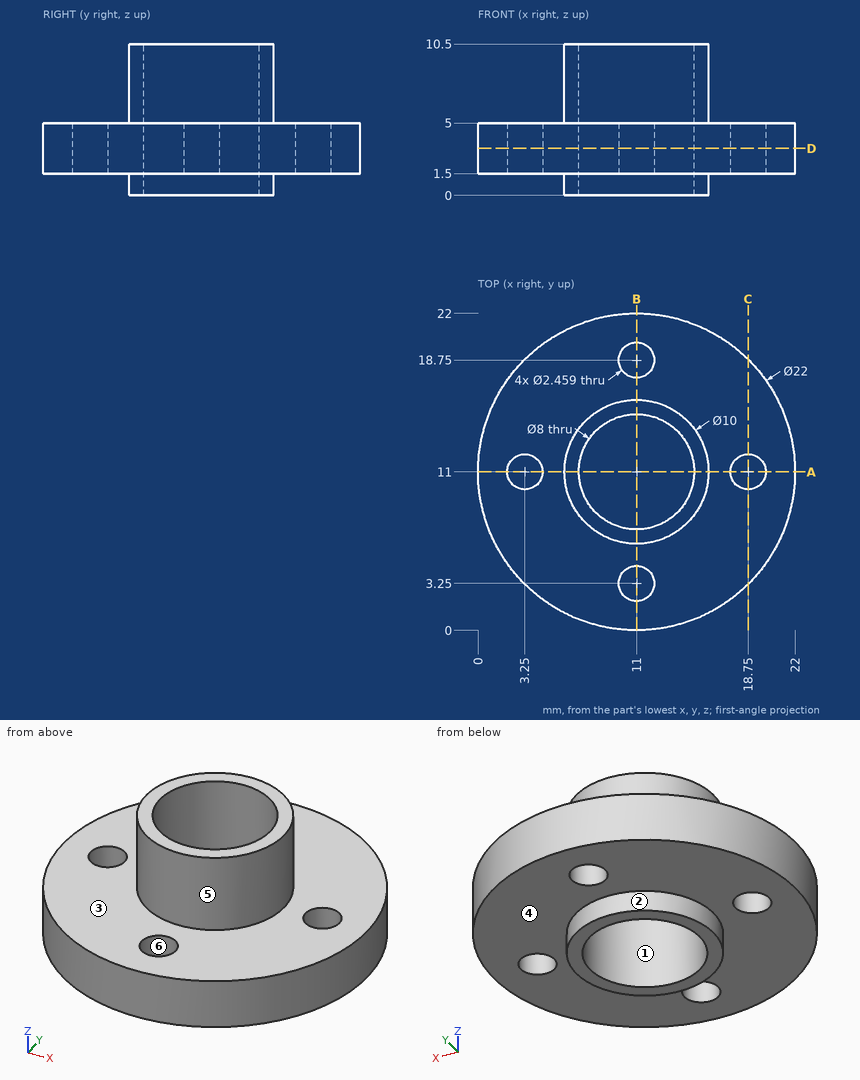
Geometry check sheet. Reference: drawing and pictorial views, mm from the part's lowest x, y, z. A direction names the side the tool comes from. Coordinates: 2 decimals unless noted, no trailing zeros. Write each loop counter-clockwise with the first axis right and the second up, starting at its lowest first coordinate (ties: lowest second). Pieces come first, ordered by that corner, then holes.
Item 1: Mould release check, pull along X, two halves, no side actions. Record for the marked faces 4, 5 and 6: released by +X, released by -X, zero draft, split by the parting line, or undercut.
Numbers:
face 4: zero draft
face 5: split by the parting line
face 6: undercut
Item 2: Access from +Z, -Z, +X, -X, +Y, -Y to the whole of each face (thin tool, end or side, straight path). Record for the marked faces 1, 2 and 3.
Numbers:
face 1: +Z, -Z
face 2: -Z
face 3: +Z
Item 3: Cross-section at D-D on z = 3.25. Record the boundary of the cut face in (x, y).
Numbers:
outline: circle Ø22 at (11, 11); hole circle Ø2.46 at (3.25, 11); hole circle Ø8 at (11, 11); hole circle Ø2.46 at (11, 3.25); hole circle Ø2.46 at (11, 18.75); hole circle Ø2.46 at (18.75, 11)
Item 4: Scan lines: probe 1 along X at (y, z) = (11, 3.7); probe 2 along Z at (x, y) = (18, 15.75); probe 3 along X at (y, z) = (11, 6.5). Record each from-to range of solid material in increasing order.
Numbers:
probe 1: x = 0 to 2.02, 4.48 to 7, 15 to 17.52, 19.98 to 22
probe 2: z = 1.5 to 5
probe 3: x = 6 to 7, 15 to 16
Item 5: Depth check by flat-ended pin: pin 1 Ø3 at (x, z) = (9, 8.5) entering from +Y; pin 2 Ø3 at (x, y) = (11, 3.25) entering from +Z; pin 3 Ø5 at (x, z) = (16, 4.5) entering from -Y. Enter the tip coordinate at first touch or a pass-through.
Numbers:
pin 1: stops at y = 15.97
pin 2: stops at z = 5
pin 3: stops at y = 0.29
Item 6: Cross-section at A-A on y = 11. Record the boundary of the cut face in (x, z), then the cut area to 3 significant figures.
Numbers:
outline: (0, 1.5) - (2.02, 1.5) - (2.02, 5) - (0, 5) - close; (4.48, 1.5) - (6, 1.5) - (6, 0) - (7, 0) - (7, 10.5) - (6, 10.5) - (6, 5) - (4.48, 5) - close; (15, 0) - (16, 0) - (16, 1.5) - (17.52, 1.5) - (17.52, 5) - (16, 5) - (16, 10.5) - (15, 10.5) - close; (19.98, 1.5) - (22, 1.5) - (22, 5) - (19.98, 5) - close
area: 45.8 mm2
Item 7: Cross-section at C-C on x = 18.75. Record the boundary of the cut face in (y, z), then the cut area to 3 significant figures.
Numbers:
outline: (3.19, 1.5) - (9.77, 1.5) - (9.77, 5) - (3.19, 5) - close; (12.23, 1.5) - (18.81, 1.5) - (18.81, 5) - (12.23, 5) - close
area: 46.0 mm2
